```python
from build123d import *

# Parameters (mm, degrees)
BOSS_EXTRUDE1_DEPTH  = 5
M5_CLEARANCE_HOLE1_D = 5.5


with BuildPart() as part:
    # Sketch1 → Boss-Extrude1 (new body, symmetric)
    with BuildSketch(Plane(origin=(0, 0, 0), x_dir=(1, 0, 0), z_dir=(0, 1, 0))):
        with BuildLine():
            ThreePointArc((0, -82.55), (82.55, 0), (0, 82.55))
            ThreePointArc((0, 82.55), (-7.5, 90.05), (0, 97.55))
            ThreePointArc((0, 97.55), (97.55, 0), (0, -97.55))
            ThreePointArc((0, -97.55), (-7.5, -90.05), (0, -82.55))
        make_face()
    extrude(amount=BOSS_EXTRUDE1_DEPTH, both=True)

    # M5 Clearance Hole1 (through all)
    with Locations(Plane(origin=(0, 5, 0), x_dir=(1, 0, 0), z_dir=(0, 1, 0))):
        with Locations((0, 90.05), (0, -90.05)):
            Hole(M5_CLEARANCE_HOLE1_D / 2)


solid = part.part
```
Part model, mm, in its own coordinate system. Give positions to 0.01 mm unless a question says otherwise; leave off trailing zeros. Write each loop counter-clockwise with the first axis right and the second up, starting at its lowest first coordinate (ties: lowest second). Pieces come first, ordered by that corner, then holes. Notation, with made-up numbers: (8, 13) -> (52, 13) arc R25 ccw to (52, 41) -> close; hole circle Ø6 at (89.25, -10.5). An arc over 180 degrees is marked (long way). Put each result on its own line as item: value. Start each with the question number.
Item 1: Cut at A-A (z = -90.05). List the corners of the cut face in (x, y).
Item 2: Cut at C-C (y = 1.5). List the corners of the cut face in (x, z).
Item 3: Cut at D-D (z = 40.5). List the corners of the cut face in (x, y).
Item 4: Pin check, flat tips, straight feed: pin 1 Ø5 at (x, y) = (16.5, -1) entering from -Z; pin 2 Ø2 at (y, z) = (1.5, -44.5) entering from +X; pin 3 Ø3 at (y, z) = (-0.5, 28.5) entering from +X; pin 4 Ø5 at (x, z) = (0, 90.05) entering from +Y. Stop position of each tip, or through.
Item 5: Wall check: L1, parallel to Z at x = 10.5, y = 1.5; L2, parallel to X at y = 1.25, z = -90.05; L3, parallel to Z at x = 67.5, y = 4.5. Give the ranges that are in metal, low to high. Write a range as [from, to].
Item 6: Cut at B-B (x = 54.5). List the corners of the cut face in (y, z).
Item 7: Pull direction Z, two halves, no side cores. Call faces 1 (the face through (84, 5, 0)), 2 (the face through (97.526, 0.07, -2.145)), 3 (the face through (-7.5, 0.1, -89.9)): pulls with the +Z half, pulls with the -Z half, needs draft (parallel to the pull), parting line crosses it, or undercut.
Answer list:
1. outline: (-7.5, -5) -> (-2.75, -5) -> (-2.75, 5) -> (-7.5, 5) -> close; (2.75, -5) -> (37.51, -5) -> (37.51, 5) -> (2.75, 5) -> close
2. outline: (0, -97.55) arc R97.55 ccw to (0, 97.55) arc R7.5 ccw to (0, 82.55) arc R82.55 cw to (0, -82.55) arc R7.5 ccw to start; hole circle Ø5.5 at (0, -90.05); hole circle Ø5.5 at (0, 90.05)
3. outline: (71.93, -5) -> (88.75, -5) -> (88.75, 5) -> (71.93, 5) -> close
4. pin 1: stops at z = -96.54
4. pin 2: stops at x = 87.31
4. pin 3: stops at x = 93.74
4. pin 4: passes through
5. L1: z = [-96.98, -81.88], [81.88, 96.98]
5. L2: x = [-7.5, -2.75], [2.75, 37.51]
5. L3: z = [-70.43, -47.52], [47.52, 70.43]
6. outline: (-5, -80.91) -> (5, -80.91) -> (5, -62) -> (-5, -62) -> close; (-5, 62) -> (5, 62) -> (5, 80.91) -> (-5, 80.91) -> close
7. face 1: needs draft
7. face 2: parting line crosses it
7. face 3: undercut
